Here's the drawing with two shaded views (mm, measured from the low corner). I have some questions. A direction names the side the tool comes from. Give positions to 0.01 mm unless a question says otherwise; leave off trailing zeros. Loops run counter-clockwise (first coordinate to the right, second up) from the corner with the lowest first, then second, coordinate; pieces in that order, holes last.
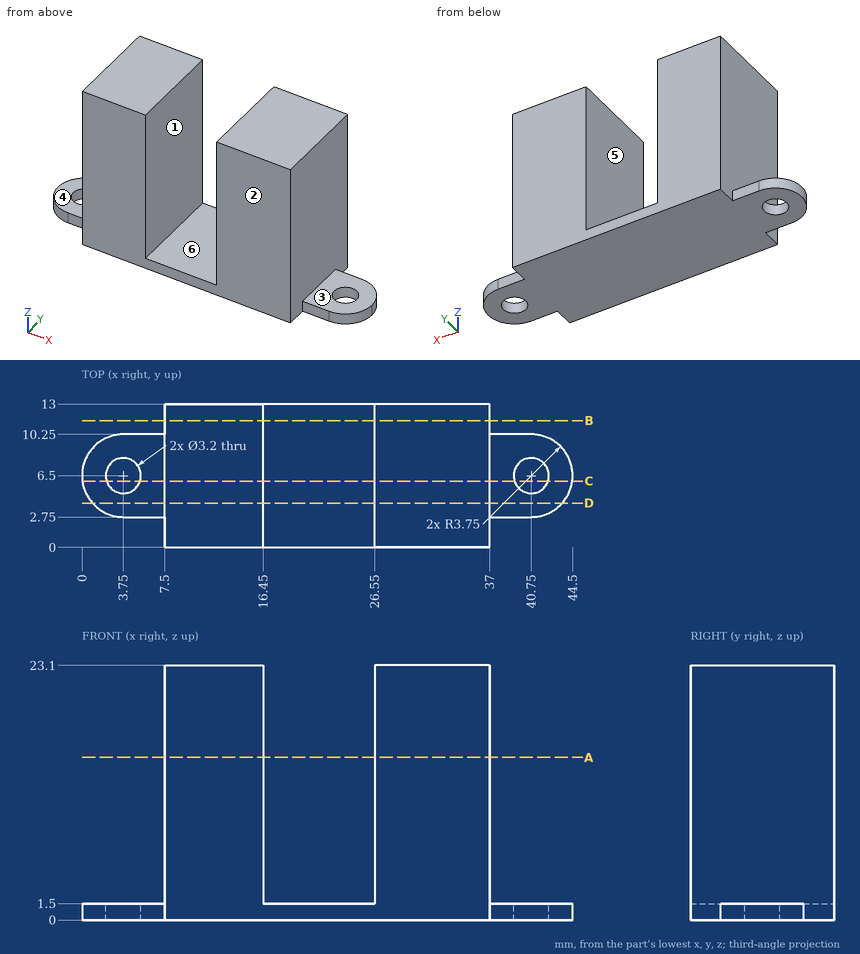
(1) Suppose I cut it at B-B on y = 11.5. List the corners of the cut face in (x, z) for me.
Returned:
outline: (7.5, 0) - (37, 0) - (37, 23.1) - (26.55, 23.1) - (26.55, 1.5) - (16.45, 1.5) - (16.45, 23.1) - (7.5, 23.1) - close
(2) Please list where these lines run through material, in increasing order: probe 1 along X at (y, z) = (6.5, 16); probe 2 along Y at (x, z) = (40.75, 0.9); probe 3 along Z at (x, y) = (17, 9).
Returned:
probe 1: x = 7.5 to 16.45, 26.55 to 37
probe 2: y = 2.75 to 4.9, 8.1 to 10.25
probe 3: z = 0 to 1.5
(3) Suppose I cut it at C-C on y = 6. List the corners of the cut face in (x, z) for me.
Returned:
outline: (0.03, 0) - (2.23, 0) - (2.23, 1.5) - (0.03, 1.5) - close; (5.27, 0) - (39.23, 0) - (39.23, 1.5) - (37, 1.5) - (37, 23.1) - (26.55, 23.1) - (26.55, 1.5) - (16.45, 1.5) - (16.45, 23.1) - (7.5, 23.1) - (7.5, 1.5) - (5.27, 1.5) - close; (42.27, 0) - (44.47, 0) - (44.47, 1.5) - (42.27, 1.5) - close
(4) Suppose I cut it at D-D on y = 4. List the corners of the cut face in (x, z) for me, plus the area to 3 significant figures.
Returned:
outline: (0.95, 0) - (43.55, 0) - (43.55, 1.5) - (37, 1.5) - (37, 23.1) - (26.55, 23.1) - (26.55, 1.5) - (16.45, 1.5) - (16.45, 23.1) - (7.5, 23.1) - (7.5, 1.5) - (0.95, 1.5) - close
area: 483 mm2
(5) Which directions (+Z, -Z, +X, -X, +Y, -Y) give clear straight access to the entire face, cutting with the end or side of a thin tool? Please do the marked faces 1, 2 and 3.
Returned:
face 1: +Z, +Y, -Y
face 2: +Z, -Z, +X, -X, -Y
face 3: +Z, +X, +Y, -Y
(6) Will these pins go through, and if not, where does the flat tip stop? P1, Ø4, axis at x = 42.5, y = 8, coming from the +Z side; P2, Ø4, axis at y = 6.5, z = 17, coming from the +X side; P3, Ø4, axis at y = 3.5, z = 13.5, coming from the -X side; P4, Ø5, axis at y = 6, z = 3, coming from the -X side.
Returned:
P1: stops at z = 1.5
P2: stops at x = 37
P3: stops at x = 7.5
P4: stops at x = 0
(7) Suppose I cut it at A-A on z = 14.75. List the corners of the cut face in (x, y) for me.
Returned:
outline: (7.5, 0) - (16.45, 0) - (16.45, 13) - (7.5, 13) - close; (26.55, 0) - (37, 0) - (37, 13) - (26.55, 13) - close
(8) Thinking about a two-plate mould opening in X: for the marked faces 4, 5 and 6, which applies, pulls with the +X half, pulls with the -X half, needs draft (parallel to the pull), parting line crosses it, or undercut?
Returned:
face 4: needs draft
face 5: undercut
face 6: undercut
